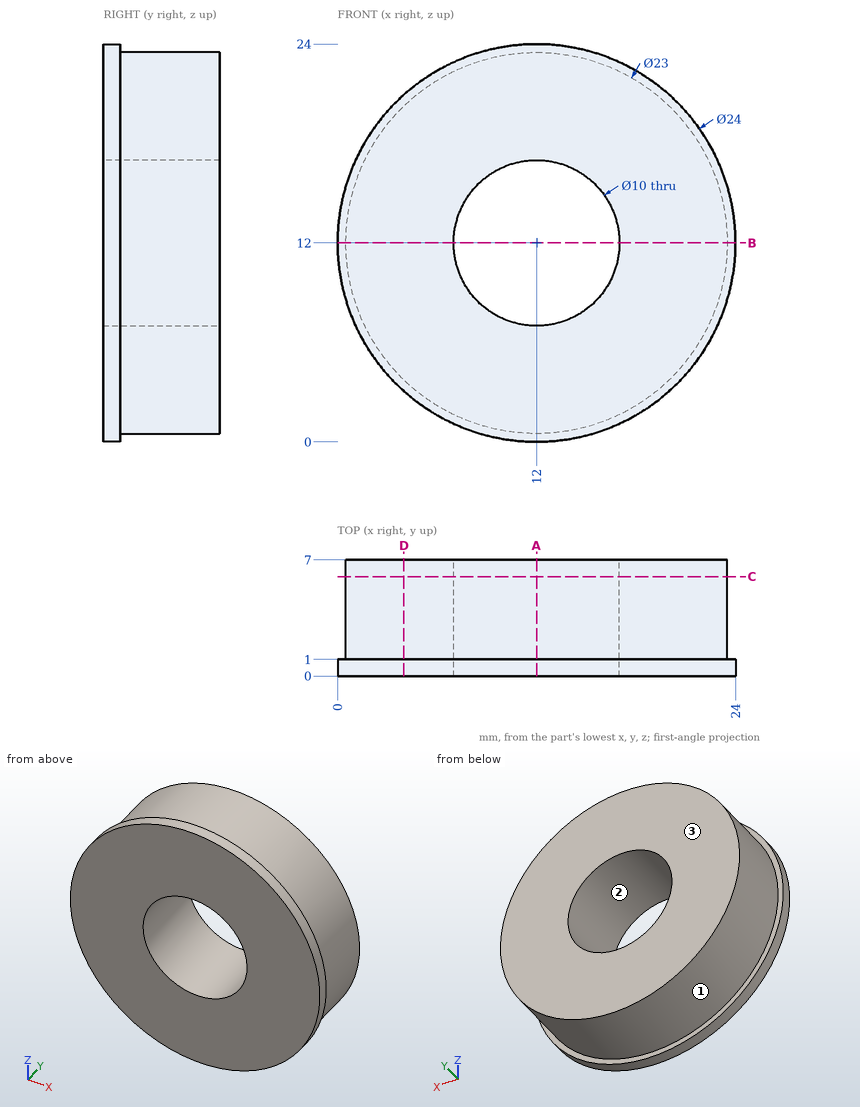
The drawing under review shows one solid part. Ordinate dimensions are in mm from its lowest x, y, z. Coordinates: 2 decimals unless noted, no trailing zeros. Write each loop counter-clockwise with the first axis right and the second up, starting at its lowest first coordinate (ties: lowest second). Pieces come first, ordered by that corner, then holes.
1) To check wall thickness, follow L1, parallel to X at y = 3.5, z = 12; L2, parallel to Z at x = 12.75, y = 5; L3, parallel to X at y = 2.75, z = 11. State the ranges of each line that lie inside material, in increasing order.
2) Mouldability with a two-part tool opening along Z and no side actions: class the marked faces 1, 2 and 3 as +Z half, -Z half, draft (parallel to the pull), parting line (faces both ways), or undercut.
3) Add section B-B (z = 12). Write out the cut boundary in (x, y), plus the area to 3 significant figures.
4) Add section D-D (x = 4). Write out the cut boundary in (y, z).
5) Add section C-C (y = 6). Write out the cut boundary in (x, z).
6) Add section A-A (x = 12). Write out the cut boundary in (y, z).
7) Insertion check: pin 1 (3 mm diameter, centred on y = 1, z = 15.5, fed in from +X); pin 2 (3 mm diameter, centred on y = 3.5, z = 19, fed in from +X). Each pin has a flat end and moves straight along its axis. Give the tip position at first contact, or say it passes through.
Check result:
1. L1: x = 0.5 to 7, 17 to 23.5
1. L2: z = 0.52 to 7.06, 16.94 to 23.48
1. L3: x = 0.54 to 7.1, 16.9 to 23.46
2. face 1: parting line
2. face 2: undercut
2. face 3: draft
3. outline: (0, 0) - (7, 0) - (7, 7) - (0.5, 7) - (0.5, 1) - (0, 1) - close; (17, 0) - (24, 0) - (24, 1) - (23.5, 1) - (23.5, 7) - (17, 7) - close
3. area: 92.0 mm2
4. outline: (0, 3.06) - (1, 3.06) - (1, 3.74) - (7, 3.74) - (7, 20.26) - (1, 20.26) - (1, 20.94) - (0, 20.94) - close
5. outline: circle Ø23 at (12, 12); hole circle Ø10 at (12, 12)
6. outline: (0, 0) - (1, 0) - (1, 0.5) - (7, 0.5) - (7, 7) - (0, 7) - close; (0, 17) - (7, 17) - (7, 23.5) - (1, 23.5) - (1, 24) - (0, 24) - close
7. pin 1: stops at x = 23.83
7. pin 2: stops at x = 22.1
